Drawing for the job (mm, zero at the part's lowest x, y, z). Round coordinates to 2 decimals unless told otherwise and drop trailing zeros. Write each loop counter-clockwise with the first axis right and the second up, starting at its lowest first coordinate (ties: lowest second). Pieces come first, ordered by that corner, then holes.
Item 1: Wall check: probe 1 along X at (y, z) = (1.5, 61); probe 2 along Z at (x, y) = (88, 0.5); probe 3 along Z at (x, y) = (50.5, 6.5). Give the ranges that are in metal, low to high.
Item 2: Band-saw the part on B-B, the plane z = 61. Write the cut outline in (x, y), then the cut area to 3 significant figures.
Item 3: Band-saw the part on C-C, the plane z = 43.5. Write the cut outline in (x, y), then the cut area to 3 significant figures.
Item 4: Band-saw the part on A-A, the plane x = 88. Write the cut outline in (y, z), then the cut area to 3 significant figures.
Item 5: Drop flat-ended pins along their axis: pin 1 Ø2.5 at (x, y) = (56.5, 5) entering from -Z; pin 2 Ø1.8 at (x, z) = (2, 61) entering from +Y; pin 3 Ø1.5 at (x, y) = (21, 4.5) entering from +Z; pin 4 Ø2.5 at (y, z) = (5.5, 20.5) entering from +X. Give the stop position or say it passes through.
Item 6: Band-saw the part on D-D, the plane y = 3.5. Write the cut outline in (x, z).
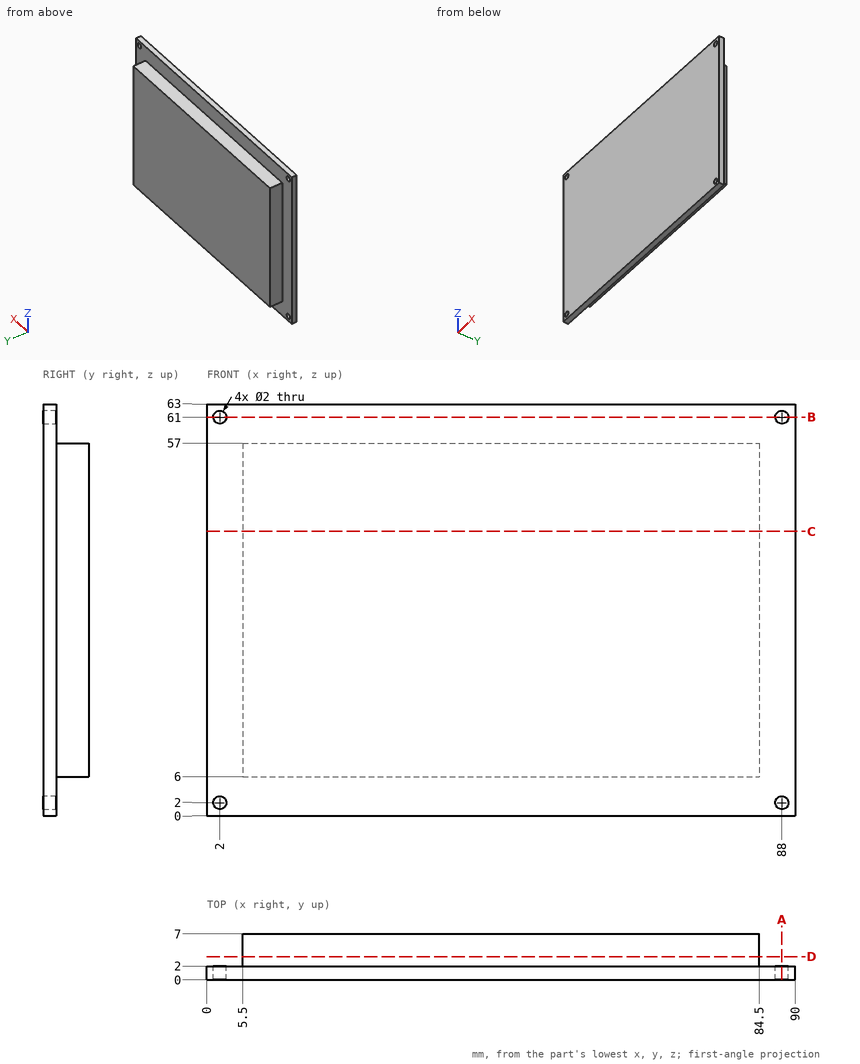
Results:
1. probe 1: x = 0 to 1, 3 to 87, 89 to 90
1. probe 2: z = 0 to 1, 3 to 60, 62 to 63
1. probe 3: z = 6 to 57
2. outline: (0, 0) - (1, 0) - (1, 2) - (0, 2) - close; (3, 0) - (87, 0) - (87, 2) - (3, 2) - close; (89, 0) - (90, 0) - (90, 2) - (89, 2) - close
2. area: 172 mm2
3. outline: (0, 0) - (90, 0) - (90, 2) - (84.5, 2) - (84.5, 7) - (5.5, 7) - (5.5, 2) - (0, 2) - close
3. area: 575 mm2
4. outline: (0, 0) - (2, 0) - (2, 1) - (0, 1) - close; (0, 3) - (2, 3) - (2, 60) - (0, 60) - close; (0, 62) - (2, 62) - (2, 63) - (0, 63) - close
4. area: 118 mm2
5. pin 1: stops at z = 6
5. pin 2: passes through
5. pin 3: stops at z = 57
5. pin 4: stops at x = 84.5
6. outline: (5.5, 6) - (84.5, 6) - (84.5, 57) - (5.5, 57) - close
